from build123d import *

# Parameters (mm, degrees)
F0_R     = 25
F0_R_2   = 12.5
F1_DEPTH = 23
F2_R     = 15.1
F3_DEPTH = 19
F4_R     = 2.25
F5_DEPTH = 25


with BuildPart() as f1:
    # F0 (on Front) → F1 (new body)
    with BuildSketch(Plane.XZ):
        Circle(F0_R)
        Circle(F0_R_2, mode=Mode.SUBTRACT)
    extrude(amount=F1_DEPTH)

    # F2 (on Front) → F3 (cut)
    with BuildSketch(Plane.XZ):
        Circle(F2_R)
    extrude(amount=F3_DEPTH, mode=Mode.SUBTRACT)

    # F4 (on face) → F5 (cut)
    with BuildSketch(Plane(origin=(0, 0, 0), x_dir=(-1, 0, 0), z_dir=(0, 1, 0))):
        with Locations((20, 0)):
            Circle(F4_R)
        with Locations((0, -20)):
            Circle(F4_R)
        with Locations((-20, 0)):
            Circle(F4_R)
        with Locations((0, 20)):
            Circle(F4_R)
    extrude(amount=-F5_DEPTH, mode=Mode.SUBTRACT)


solid = f1.part
Geometry: final body of the model. Coordinates: model frame, mm. A direction names the side the tool comes from. Round coordinates to 2 decimals unless told otherwise and drop trailing zeros. Order: outer loops, then holes, each group sorted by start corner. A loop starts at its lowest first (then second) coordinate and runs counter-clockwise, first axis right, second up. Notation, with made-up numbers: (22.5, 5.25) -> (70.5, 5.25) arc R33 cw to (70.5, 43.25) -> close; hole circle Ø4 at (35, 42.25). An arc over 180 degrees is marked (long way). Put each result on its own line as item: value. Start each with the question number.
Q1. Section C-C on z = -20. Return the cut outline in (x, y), and give its area (4 significant figures).
Q2. Pull-direction query (Z, two-part tool) for faces 1 (the flat face through (11, 0, -11)), 2 (the cylindrical face through (23.846, -11.339, 7.509)), 3 (the flat face through (-5.7, -19, 11.3)); classes: +Z half, -Z half, draft (parallel to the pull), parting line (faces both ways), or undercut.
Q3. Section D-D on y = -5.5. Return the cut outline in (x, z), and give its area (3 significant figures).
Q4. First-contact query: pin 1 (1.5 mm diameter, centred on y = -18, z = -13.5, fed in from -X); pin 2 (2.5 mm diameter, centred on x = 20, z = 0, fed in from +Y); pin 3 (6 mm diameter, centred on y = -11.5, z = -18, fed in from +X); pin 4 (4 mm diameter, centred on x = 3.5, y = -2.5, fed in from +Z). Flat tips, straight axial feed; report the tip coordinate or a pass-through.
Q5. Section A-A on z = 0. Return the cut outline in (x, y), and give its area (3 significant figures).
Q6. Section B-B on x = -20. Return the cut outline in (y, z).
Q7. Reachability of faces 4 (the cylindrical face through (0.488, -11.339, 17.804)), 5 (the cylindrical face through (-3.27, -9.37, -14.74)) from +Z, -Z, +X, -X, +Y, -Y: full face, straight path, thin tool, end or side. Return the list, or none.
Q8. Line query: probe 1 along Z at (x, y) = (0, -14.5); probe 2 along X at (y, z) = (-15.5, -2); probe 3 along Z at (x, y) = (20.5, -17). Output: solid intervals per line, ascending.
Ans:
1. outline: (-15, -23) -> (-2.25, -23) -> (-2.25, 0) -> (-15, 0) -> close; (2.25, -23) -> (15, -23) -> (15, 0) -> (2.25, 0) -> close
1. area: 586.5 mm2
2. face 1: draft
2. face 2: parting line
2. face 3: undercut
3. outline: circle Ø50 at (0, 0); hole circle Ø4.5 at (-20, 0); hole circle Ø30.2 at (0, 0); hole circle Ø4.5 at (0, -20); hole circle Ø4.5 at (0, 20); hole circle Ø4.5 at (20, 0)
3. area: 1,180 mm2
4. pin 1: stops at x = -21.5
4. pin 2: passes through
4. pin 3: stops at x = 20
4. pin 4: stops at z = 24.95
5. outline: (-25, -23) -> (-22.25, -23) -> (-22.25, 0) -> (-25, 0) -> close; (-17.75, -23) -> (-12.5, -23) -> (-12.5, -19) -> (-15.1, -19) -> (-15.1, 0) -> (-17.75, 0) -> close; (12.5, -23) -> (17.75, -23) -> (17.75, 0) -> (15.1, 0) -> (15.1, -19) -> (12.5, -19) -> close; (22.25, -23) -> (25, -23) -> (25, 0) -> (22.25, 0) -> close
5. area: 269 mm2
6. outline: (-23, -15) -> (0, -15) -> (0, -2.25) -> (-23, -2.25) -> close; (-23, 2.25) -> (0, 2.25) -> (0, 15) -> (-23, 15) -> close
7. face 4: +Y, -Y
7. face 5: +Y
8. probe 1: z = -25 to -22.25, -17.75 to -15.1, 15.1 to 17.75, 22.25 to 25
8. probe 2: x = -24.92 to -21.03, -18.97 to -14.97, 14.97 to 18.97, 21.03 to 24.92
8. probe 3: z = -14.31 to -2.19, 2.19 to 14.31
